```python
from build123d import *

# Parameters (mm, degrees)
BOSS_EXTRUDE1_DEPTH = 4
SKETCH1_3_R         = 1
CUT_EXTRUDE2_DEPTH  = 4
SKETCH1_4_R         = 2.5
BOSS_EXTRUDE2_DEPTH = 4
SKETCH1_5_R         = 2
BOSS_EXTRUDE3_DEPTH = 9
CHAMFER1_SIZE       = 0.5
FILLET1_R           = 0.5
SKETCH2_R           = 2
CUT_EXTRUDE3_DEPTH  = 2.5


with BuildPart() as part:
    # Sketch1 → Boss-Extrude1 (new body)
    with BuildSketch(Plane(origin=(0, 0, 0), x_dir=(0, 0, -1), z_dir=(1, 0, 0))):
        with BuildLine():
            Line((-5.921359641, 5), (5.921359641, 5))
            ThreePointArc((5.921359641, 5), (0, -7.75), (-5.921359641, 5))
        make_face()
    extrude(amount=BOSS_EXTRUDE1_DEPTH)

    # Sketch1<3> → Cut-Extrude2 (cut)
    with BuildSketch(Plane(origin=(0, 0, 0), x_dir=(0, 0, -1), z_dir=(1, 0, 0))):
        with Locations((-5, 0)):
            Circle(SKETCH1_3_R)
        with Locations((5, 0)):
            Circle(SKETCH1_3_R)
        with Locations((0, -5)):
            Circle(SKETCH1_3_R)
    extrude(amount=CUT_EXTRUDE2_DEPTH, mode=Mode.SUBTRACT)

    # Sketch1<4> → Boss-Extrude2 (add)
    with BuildSketch(Plane(origin=(0, 0, 0), x_dir=(0, 0, -1), z_dir=(1, 0, 0))):
        Circle(SKETCH1_4_R)
    extrude(amount=-BOSS_EXTRUDE2_DEPTH)

    # Sketch1<5> → Boss-Extrude3 (add)
    with BuildSketch(Plane(origin=(0, 0, 0), x_dir=(0, 0, -1), z_dir=(1, 0, 0))):
        Circle(SKETCH1_5_R)
    extrude(amount=-BOSS_EXTRUDE3_DEPTH)

    # Chamfer1
    chamfer1_edges = [part.edges().sort_by_distance(p)[0] for p in [
        (-9, 0, 2),
    ]]
    chamfer(chamfer1_edges, length=CHAMFER1_SIZE)

    # Fillet1
    fillet1_edges = [part.edges().sort_by_distance(p)[0] for p in [
        (2, 5, 5.921359641),
        (2, 5, -5.921359641),
    ]]
    fillet(fillet1_edges, radius=FILLET1_R)

    # Sketch2 → Cut-Extrude3 (cut)
    with BuildSketch(Plane(origin=(4, 0, 0), x_dir=(0, 0, -1), z_dir=(1, 0, 0))):
        with Locations((-5, 0)):
            Circle(SKETCH2_R)
        with Locations((5, 0)):
            Circle(SKETCH2_R)
        with Locations((0, -5)):
            Circle(SKETCH2_R)
    extrude(amount=-CUT_EXTRUDE3_DEPTH, mode=Mode.SUBTRACT)


solid = part.part
```
Design review of the part built by this model. Coordinates are the model's own, in mm. A direction names the side the tool comes from. Coordinates: 2 decimals unless noted, no trailing zeros. Loops run counter-clockwise (first coordinate to the right, second up) from the corner with the lowest first, then second, coordinate; pieces in that order, holes last.
Q1. The part is to be moulded in two halves that separate along Z. For faces 4 (the face through (1.5, -1, 4)), 5 (the face through (0.7, -0.6, 5.8)), 6 (the face through (-6, -2, 0)), 7 (the face through (-9, 0, 0)), say which applies: +Z half, -Z half, draft (parallel to the pull), parting line (faces both ways), or undercut.
Reported:
face 4: undercut
face 5: undercut
face 6: parting line
face 7: draft
Q2. Tool access review of faces 1 (the face through (2.8, -1.2, 6.6)), 2 (the face through (2, 5, 0)), 3 (the face through (-1.97, -2.44, 0.54)): name each direction out of +Z, -Z, +X, -X, +Y, -Y from which nothing blocks a thin tool from reaching the whole face with its end or side.
Reported:
face 1: +X
face 2: +Z, -Z, +X, -X, +Y
face 3: -X
Q3. We need section C-C on z = 4.75. State the section outline as (x, y) points.
Reported:
outline: (0, -6.12) - (4, -6.12) - (4, -1.98) - (1.5, -1.98) - (1.5, -0.97) - (0, -0.97) - close; (0, 0.97) - (1.5, 0.97) - (1.5, 1.98) - (4, 1.98) - (4, 5) - (0, 5) - close
Q4. We need section D-D on y = -5. State the section outline as (x, z) points, and give its area (3 significant figures).
Reported:
outline: (0, -5.92) - (4, -5.92) - (4, -2) - (1.5, -2) - (1.5, -1) - (0, -1) - close; (0, 1) - (1.5, 1) - (1.5, 2) - (4, 2) - (4, 5.92) - (0, 5.92) - close
area: 34.4 mm2
Q5. We need section B-B on x = 1.25. State the section outline as (y, z) points.
Reported:
outline: (4.81, -6.08) arc R0.5 ccw to (5, -5.68) - (5, 5.68) arc R0.5 ccw to (4.81, 6.08) arc R7.75 ccw (long way) to start; hole circle Ø2 at (-5, 0); hole circle Ø2 at (0, -5); hole circle Ø2 at (0, 5)
Q6. To check wall thickness, follow line 1 (Z direction, x = 1, y = 0); line 2 (Y direction, x = 3.4, z = 0); line 3 (Y direction, x = 1.05, z = 0). State the ranges of each line that lie inside material, in increasing order.
Reported:
line 1: z = -7.75 to -6, -4 to 4, 6 to 7.75
line 2: y = -7.75 to -7, -3 to 5
line 3: y = -7.75 to -6, -4 to 5
Q7. We need section A-A on y = 0. State how many separate pieces and enclosed holes the cut face has, and give its area (4 significant figures).
Reported:
separate pieces: 3
enclosed holes: 0
area: 75.75 mm2
Q8. For pin 1 (2.5 mm diameter, centred on y = 0, z = 5, fed in from -X); pin 2 (2.5 mm diameter, centred on y = 0, z = -5, fed in from +X); pin 3 (1.6 mm diameter, centred on y = -5, z = 0, fed in from +X); pin 4 (6.5 mm diameter, centred on y = 0, z = -5, fed in from -X), all flat-tipped, find the tip position at first contact; note any pin that passes through.
Reported:
pin 1: stops at x = 0
pin 2: stops at x = 1.5
pin 3: passes through
pin 4: stops at x = -8.75
